The listing builds one solid part. Answer for the finished solid, in the listing's coordinates (mm). A direction names the side the tool comes from. Give positions to 0.01 mm unless a question says otherwise; leave off trailing zeros. Write each loop counter-clockwise with the first axis right and the second up, starting at its lowest first coordinate (ties: lowest second). Pieces come first, ordered by that corner, then holes. Notation, with made-up numbers: (4, 16) - (18, 16) arc R27 cw to (18, 41) - close; hole circle Ø10 at (60.25, -8.75). An arc over 180 degrees is marked (long way). Write each question's results on one line, items separated by ' | '. Start each with the question number.
Q1. Find the intervals of material crossed by probe 1 along Y at (x, z) = (4.35, 3); probe 2 along X at (y, z) = (0.5, 5.25); probe 3 along X at (y, z) = (7.5, -1.45), in increasing order.
Q2. Flat-ended cylindrical pins translate along their axes: pin 1 Ø1.6 at (x, z) = (4.5, 1.5) entering from +Y; pin 2 Ø4 at (x, y) = (3.5, 7.5) entering from +Z; pin 3 Ø4 at (x, z) = (-0.5, 4.5) entering from -Y; pin 4 Ø1 at (x, z) = (3.5, 1.5) entering from -Y. Find the tip coordinate at first contact, or state that the pin passes through.
Q3. Section A-A (y = -7.5) is taken. Determine the outline of the cut face in (x, z) (3 decimals), plus the area to 3 significant figures.
Q4. For a pull along X with two mould halves and no side action, classify faces 3 (the face through (-4.01, 2.14, 5.1)), 4 (the face through (-4.43, 9.4, -1.01)), 5 (the face through (-3, 1, 1)), 6 (the face through (3, 1, 1)) as pulls with the +X half, pulls with the -X half, needs draft (parallel to the pull), parting line crosses it, or undercut.
Q5. Section D-D (z = 2.5) is taken. State how many separate pieces and enclosed holes the cut face has, plus the area to 3 significant figures.
Q6. For faces 1 (the face through (4, 3, 2)), 2 (the face through (3.986, -3.301, 0.285)), determine the directions among +Z, -Z, +X, -X, +Y, -Y from which every point of the face is accessible in a straight line to the end or side of a thin tool.
```python
from build123d import *

# Parameters (mm, degrees)
SKETCH1_W                       = 20
SKETCH1_H                       = 10
BOSS_EXTRUDE1_DEPTH             = 2
SKETCH2_W                       = 6
SKETCH2_H                       = 2
BOSS_EXTRUDE2_DEPTH             = 6
FILLET1_R                       = 3
F_4_0MM_DOWEL_HOLE1_D           = 4
F_4_0MM_DOWEL_HOLE1_CSINK_D     = 4.05
F_4_0MM_DOWEL_HOLE1_CSINK_ANGLE = 90
F_2_0MM_DOWEL_HOLE1_D           = 2
F_2_0MM_DOWEL_HOLE1_CSINK_D     = 2.05
F_2_0MM_DOWEL_HOLE1_CSINK_ANGLE = 90
FILLET2_R                       = 1
FILLET3_R                       = 2


with BuildPart() as part:
    # Sketch1 → Boss-Extrude1 (new body)
    with BuildSketch(Plane(origin=(0, 0, 0), x_dir=(0, 1, 0), z_dir=(0, 0, 1))):
        Rectangle(SKETCH1_W, SKETCH1_H)
    extrude(amount=-BOSS_EXTRUDE1_DEPTH)

    # Sketch2 → Boss-Extrude2 (add)
    with BuildSketch(Plane(origin=(0, 0, 0), x_dir=(0, 1, 0), z_dir=(0, 0, 1))):
        with Locations((0, 4)):
            Rectangle(SKETCH2_W, SKETCH2_H)
        with Locations((0, -4)):
            Rectangle(SKETCH2_W, SKETCH2_H)
    extrude(amount=BOSS_EXTRUDE2_DEPTH)

    # Fillet1
    fillet1_edges = [part.edges().sort_by_distance(p)[0] for p in [
        (4, 3, 6),
        (4, -3, 6),
        (-4, 3, 6),
        (-4, -3, 6),
    ]]
    fillet(fillet1_edges, radius=FILLET1_R - 0.0001)  # a hair under: the kernel refuses the full size

    # Ø4.0mm Dowel Hole1 (through all)
    with Locations(Plane.YZ.offset(5)):
        with Locations((0, 3)):
            CounterSinkHole(F_4_0MM_DOWEL_HOLE1_D / 2, F_4_0MM_DOWEL_HOLE1_CSINK_D / 2, counter_sink_angle=F_4_0MM_DOWEL_HOLE1_CSINK_ANGLE)

    # Ø2.0mm Dowel Hole1 (through all)
    with Locations(Plane(origin=(0, 0, 0), x_dir=(0, 1, 0), z_dir=(0, 0, 1))):
        with Locations((7.5, -3), (-7.5, 3), (-7.5, -3), (7.5, 3)):
            CounterSinkHole(F_2_0MM_DOWEL_HOLE1_D / 2, F_2_0MM_DOWEL_HOLE1_CSINK_D / 2, counter_sink_angle=F_2_0MM_DOWEL_HOLE1_CSINK_ANGLE)

    # Fillet2
    fillet2_edges = [part.edges().sort_by_distance(p)[0] for p in [
        (-4, -3, 0),
        (-4, 3, 0),
        (4, -3, 0),
        (4, 3, 0),
    ]]
    fillet(fillet2_edges, radius=FILLET2_R)

    # Fillet3
    fillet3_edges = [part.edges().sort_by_distance(p)[0] for p in [
        (-5, -10, -1),
        (-5, 10, -1),
        (5, 10, -1),
        (5, -10, -1),
    ]]
    fillet(fillet3_edges, radius=FILLET3_R)


solid = part.part
```
Answers below:
1) probe 1: y = -3 to -2, 2 to 3 | probe 2: x = -5 to -3, 3 to 5 | probe 3: x = -5 to -4, -2 to 2, 4 to 5
2) pin 1: stops at y = 3.05 | pin 2: stops at z = 0 | pin 3: passes through | pin 4: stops at y = -3
3) outline: (-5, -2) - (-4, -2) - (-4, -0.025) - (-4.025, 0) - (-5, 0) - close; (-2, -2) - (2, -2) - (2, -0.025) - (1.975, 0) - (-1.975, 0) - (-2, -0.025) - close; (4, -2) - (5, -2) - (5, 0) - (4.025, 0) - (4, -0.025) - close | area: 12.0 mm2
4) face 3: needs draft | face 4: pulls with the -X half | face 5: undercut | face 6: undercut
5) separate pieces: 4 | enclosed holes: 0 | area: 8.51 mm2
6) face 1: +Z, +X, -X, +Y | face 2: +Z, +X, -X, -Y
